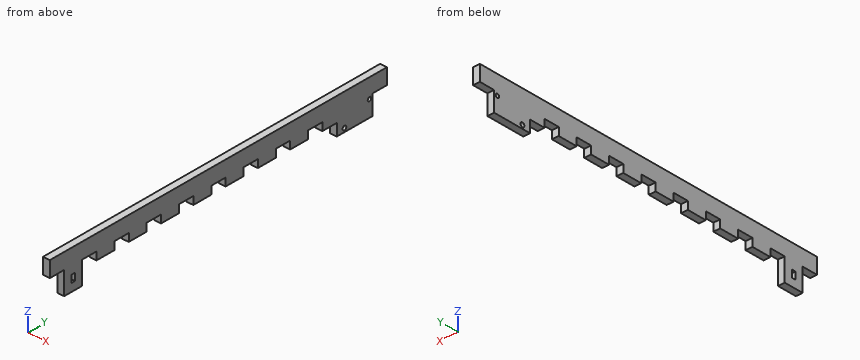
```python
from build123d import *

# Parameters (mm, degrees)
BOSS_EXTRUDE1_DEPTH = 5.588
SKETCH2_W           = 15.9999934
SKETCH2_H           = 31.75
SKETCH2_R           = 1.55
SKETCH2_R_2         = 1.7
BOSS_EXTRUDE2_DEPTH = 5.588
SKETCH2_4_R         = 1.55
CUT_EXTRUDE1_DEPTH  = 6.588


with BuildPart() as part:
    # Sketch1 → Boss-Extrude1 (new body)
    with BuildSketch(Plane(origin=(0, 0, 0), x_dir=(0, 0, -1), z_dir=(1, 0, 0))):
        Polygon((3.175, 120.65), (9.525, 120.65), (9.525, 136.525), (3.175, 136.525), (3.175, 149.225), (-9.525, 149.225), (-9.525, -149.225), (3.175, -149.225), (3.175, -136.525), (9.525, -136.525), (9.525, -120.65), (3.175, -120.65), (3.175, -107.95), (9.525, -107.95), (9.525, -92.075), (3.175, -92.075), (3.175, -79.375), (9.525, -79.375), (9.525, -63.5), (3.175, -63.5), (3.175, -50.8), (9.525, -50.8), (9.525, -34.925), (3.175, -34.925), (3.175, -22.225), (9.525, -22.225), (9.525, -6.35), (3.175, -6.35), (3.175, 6.35), (9.525, 6.35), (9.525, 22.225), (3.175, 22.225), (3.175, 34.925), (9.525, 34.925), (9.525, 50.8), (3.175, 50.8), (3.175, 63.5), (9.525, 63.5), (9.525, 79.375), (3.175, 79.375), (3.175, 92.075), (9.525, 92.075), (9.525, 107.95), (3.175, 107.95), align=None)
    extrude(amount=BOSS_EXTRUDE1_DEPTH)

    # Sketch2 → Boss-Extrude2 (add)
    with BuildSketch(Plane(origin=(5.588, 0, 0), x_dir=(0, 0, -1), z_dir=(1, 0, 0))):
        Polygon((21.717, -120.65), (9.525, -120.65), (9.525, -127), (15.367, -127), (15.367, -130.175), (9.525, -130.175), (9.525, -136.525), (21.717, -136.525), align=None)
        with Locations((11.1749967, 120.65)):
            Rectangle(SKETCH2_W, SKETCH2_H)
        with Locations((5.9749992, 133.7250056)):
            Circle(SKETCH2_R, mode=Mode.SUBTRACT)
        with Locations((16.2749992, 111.5250056)):
            Circle(SKETCH2_R_2, mode=Mode.SUBTRACT)
    extrude(amount=-BOSS_EXTRUDE2_DEPTH)

    # Sketch2<4> → Cut-Extrude1 (cut, through all)
    with BuildSketch(Plane(origin=(5.588, 0, 0), x_dir=(0, 0, -1), z_dir=(1, 0, 0))):
        with Locations((5.9749992, 133.7250056)):
            Circle(SKETCH2_4_R)
    extrude(amount=-CUT_EXTRUDE1_DEPTH, mode=Mode.SUBTRACT)


solid = part.part
```
Can you work these out from the model? Positions are in its coordinate system, mm. Coordinates: 2 decimals unless noted, no trailing zeros. Loops run counter-clockwise (first coordinate to the right, second up) from the corner with the lowest first, then second, coordinate; pieces in that order, holes last.
1) Imagine slicing it at B-B on y = -15. List the corners of the cut face in (x, z) for me (3 decimals), plus the area to 3 significant figures.
2) I need wall thicknesses on probe 1 along Y at (x, z) = (0.6, -11) (3 decimals); probe 2 along Y at (x, z) = (2, -16) (3 decimals); probe 3 along Y at (x, z) = (3.75, -19) (3 decimals). Which ranges of each line are inside material? Lowest first, please.
3) Imagine slicing it at A-A on z = -12. List the corners of the cut face in (x, y) for me (3 decimals).
4) For pin 1 (3 mm diameter, centred on x = 4, z = -14, fed in from -Y) (3 decimals); pin 2 (1.7 mm diameter, centred on x = 2.5, y = -13, fed in from -Z) (3 decimals); pin 3 (3 mm diameter, centred on x = 3, y = -26, fed in from -Z) (3 decimals); pin 4 (8 mm diameter, centred on y = 29.5, z = 5.5, fed in from -X), each with a flat end and sliding along its axis, tell me the tip position at first contact or that it passes through.
5) Imagine slicing it at C-C on x = 4.6. State how many separate pieces and enclosed holes the cut face has, plus the area to 3 significant figures.
6) Imagine slicing it at D-D on y = 89. List the corners of the cut face in (x, z) for me (3 decimals).
Completed:
1. outline: (0, -9.525) - (5.588, -9.525) - (5.588, 9.525) - (0, 9.525) - close
1. area: 106 mm2
2. probe 1: y = -136.525 to -130.175, -127 to -120.65, 104.775 to 136.525
2. probe 2: y = -136.525 to -120.65, 104.775 to 109.847, 113.203 to 136.525
2. probe 3: y = -136.525 to -120.65, 104.775 to 136.525
3. outline: (0, -136.525) - (5.588, -136.525) - (5.588, -130.175) - (0, -130.175) - close; (0, -127) - (5.588, -127) - (5.588, -120.65) - (0, -120.65) - close; (0, 104.775) - (5.588, 104.775) - (5.588, 136.525) - (0, 136.525) - close
4. pin 1: stops at y = -136.525
4. pin 2: stops at z = -9.525
4. pin 3: stops at z = -3.175
4. pin 4: stops at x = 0
5. separate pieces: 1
5. enclosed holes: 3
5. area: 5,340 mm2
6. outline: (0, -3.175) - (5.588, -3.175) - (5.588, 9.525) - (0, 9.525) - close
